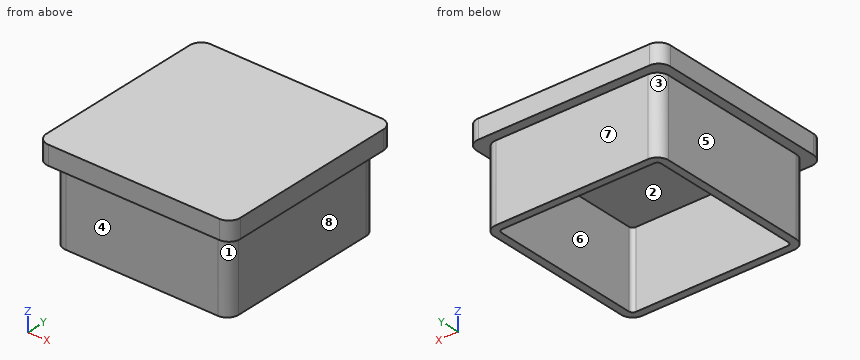
from build123d import *

# Parameters (mm, degrees)
F1_DEPTH = 5
F3_DEPTH = 20


with BuildPart() as f1:
    # F0 (on Top) → F1 (new body)
    with BuildSketch(Plane.XY):
        with BuildLine():
            ThreePointArc((-25.5, -22.5), (-24.62132, -24.62132), (-22.5, -25.5))
            Line((-22.5, -25.5), (22.5, -25.5))
            ThreePointArc((22.5, -25.5), (24.62132, -24.62132), (25.5, -22.5))
            Line((25.5, -22.5), (25.5, 22.5))
            ThreePointArc((25.5, 22.5), (24.62132, 24.62132), (22.5, 25.5))
            Line((22.5, 25.5), (-22.5, 25.5))
            ThreePointArc((-22.5, 25.5), (-24.62132, 24.62132), (-25.5, 22.5))
            Line((-25.5, 22.5), (-25.5, -22.5))
        make_face()
    extrude(amount=F1_DEPTH)

    # F2 (on face) → F3 (join)
    with BuildSketch(Plane(origin=(0, 0, 0), x_dir=(1, 0, 0), z_dir=(0, 0, -1))):
        with BuildLine():
            ThreePointArc((-23, -20), (-22.12132, -22.12132), (-20, -23))
            Line((-20, -23), (20, -23))
            ThreePointArc((20, -23), (22.12132, -22.12132), (23, -20))
            Line((23, -20), (23, 20))
            ThreePointArc((23, 20), (22.12132, 22.12132), (20, 23))
            Line((20, 23), (-20, 23))
            ThreePointArc((-20, 23), (-22.12132, 22.12132), (-23, 20))
            Line((-23, 20), (-23, -20))
        make_face()
        with BuildLine():
            ThreePointArc((20, 21), (20.707107, 20.707107), (21, 20))
            Line((21, 20), (21, -20))
            ThreePointArc((21, -20), (20.707107, -20.707107), (20, -21))
            Line((20, -21), (-20, -21))
            ThreePointArc((-20, -21), (-20.707107, -20.707107), (-21, -20))
            Line((-21, -20), (-21, 20))
            ThreePointArc((-21, 20), (-20.707107, 20.707107), (-20, 21))
            Line((-20, 21), (20, 21))
        make_face(mode=Mode.SUBTRACT)
    extrude(amount=F3_DEPTH)


solid = f1.part
Could you check a few things on this model? Use its own coordinates, in mm. Face numbers are marked on the shaded views. A direction names the side the tool comes from. Coordinates: 2 decimals unless noted, no trailing zeros. Order: outer loops, then holes, each group sorted by start corner. A loop starts at its lowest first (then second) coordinate and runs counter-clockwise, first axis right, second up. Notation, with made-up numbers: (60, -12.75) -> (87, -12.75) arc R16 ccw to (87, 3.25) -> close; hole circle Ø6 at (-22, -18.5). An arc over 180 degrees is marked (long way). One line per question, with ' | ' between items.
Q1. Thinking about a two-plate mould opening in X: for the marked faces 6, 7 and 8, which applies, pulls with the +X half, pulls with the -X half, needs draft (parallel to the pull), parting line crosses it, or undercut?
Return value:
face 6: undercut | face 7: needs draft | face 8: pulls with the +X half
Q2. On a 3-axis mill with a long thin cutter (end or side, diameter ignored), from which of +Z, -Z, +X, -X, +Y, -Y can I reach the whole of each face in a straight line? I mean the marked faces 1, 2, 3, 4 and 5. Say none if no direction works.
Return value:
face 1: -Z, +X, -Y | face 2: -Z | face 3: -Z, -X, +Y | face 4: -Z, +X, -X, -Y | face 5: -Z, -X, +Y, -Y
Q3. I'm going to push flat-ended pins straight in: P1, Ø12.5, axis at x = 8.5, y = -6.5, coming from the -Z side; P2, Ø6, axis at y = -1, z = -5, coming from the +X side; P3, Ø6, axis at x = -6, z = -8.5, coming from the -Y side. Where does each tip first touch, or does it pass through?
Return value:
P1: z = 0 | P2: x = 23 | P3: y = -23
Q4. Imagine slicing it at A-A on z = -1. Please give me the cut outline in (x, y).
Return value:
outline: (-23, -20) arc R3 ccw to (-20, -23) -> (20, -23) arc R3 ccw to (23, -20) -> (23, 20) arc R3 ccw to (20, 23) -> (-20, 23) arc R3 ccw to (-23, 20) -> close; hole (-21, -20) arc R1 ccw to (-20, -21) -> (20, -21) arc R1 ccw to (21, -20) -> (21, 20) arc R1 ccw to (20, 21) -> (-20, 21) arc R1 ccw to (-21, 20) -> close
Q5. Imagine slicing it at B-B on y = 13.5. Please give me the cut outline in (x, z), and give its area (3 significant figures).
Return value:
outline: (-25.5, 0) -> (-23, 0) -> (-23, -20) -> (-21, -20) -> (-21, 0) -> (21, 0) -> (21, -20) -> (23, -20) -> (23, 0) -> (25.5, 0) -> (25.5, 5) -> (-25.5, 5) -> close | area: 335 mm²
Q6. If I drill on L1, parallel to X at y = 15, z = -5.25; L2, parallel to Z at x = 13.5, y = -8.5, over which ranges is the centre line in solid material (lowest first)?
Return value:
L1: -23 to -21, 21 to 23 | L2: 0 to 5
